from build123d import *

# Parameters (mm, degrees)
SKETCH_3_R          = 6
CUT_EXTRUDE_1_DEPTH = 1
CHAMFER_1_SIZE      = 1
CHAMFER_1_SIZE2     = 0.363970234
CHAMFER_2_SIZE      = 0.5
CHAMFER_2_SIZE2     = 0.181985117


with BuildPart() as part:
    # Эскиз1 → Повернуть1 (revolve)
    with BuildSketch(Plane.XY):
        Polygon((0, 0), (0, 5), (5, 5), (5, 0), (9, 0), (9, -3), (0, -3), align=None)
    revolve(axis=Axis((0, 0, 0), (0, 1, 0)))

    # Эскиз3 → Вырез-Вытянуть1 (cut)
    with BuildSketch(Plane.XZ.offset(3)):
        Circle(SKETCH_3_R)
    extrude(amount=-CUT_EXTRUDE_1_DEPTH, mode=Mode.SUBTRACT)

    # Фаска1
    chamfer_1_edges = [part.edges().sort_by_distance(p)[0] for p in [
        (-6, -3, 0),
    ]]
    chamfer_1_side = [part.faces().sort_by_distance(p)[0] for p in [
        (-8.745441559, -3, 0),
    ]]
    chamfer(chamfer_1_edges, length=CHAMFER_1_SIZE, length2=CHAMFER_1_SIZE2, reference=chamfer_1_side[0])

    # Фаска2
    chamfer_2_edges = [part.edges().sort_by_distance(p)[0] for p in [
        (-9, -3, 0),
    ]]
    chamfer_2_side = [part.faces().sort_by_distance(p)[0] for p in [
        (-9, -1.5, 0),
    ]]
    chamfer(chamfer_2_edges, length=CHAMFER_2_SIZE, length2=CHAMFER_2_SIZE2, reference=chamfer_2_side[0])


solid = part.part
Verification items for the finished model (mm, model axes). A direction names the side the tool comes from. Coordinates: 2 decimals unless noted, no trailing zeros. Write each loop counter-clockwise with the first axis right and the second up, starting at its lowest first coordinate (ties: lowest second). Pieces come first, ordered by that corner, then holes. Notation, with made-up numbers: M 73.5,89 L 82.5,89 A31 ccw 82.5,122 Z; hole C 71,55 d7. An arc over 180 degrees is marked long. Use a Markdown table: item, result.
Q1. Set-up check for faces 4 (the face through (0, -2, 0)), 5 (the face through (-3, -3, -7)), 6 (the face through (-1.08, 2.46, 4.88)): record each of +Z, -Z, +X, -X, +Y, -Y from which the full face is reachable in a straight line by a thin tool's end or side.
Reply:
| item | result |
|---|---|
| face 4 | -Y |
| face 5 | +Z, -Z, +X, -X, -Y |
| face 6 | +Y |
Q2. Sectioned sample at C-C, the plane y = -1.25. Record the boundary of the cut face in (x, z).
Reply:
| item | result |
|---|---|
| outline | C 0,0 d18 |
Q3. Draft check along X on faces 1 (the face through (0, 5, 0)), 2 (the face through (-5.994, -2.322, 0.264)), 3 (the face through (-1.172, -1.268, -8.923)). Enter one of: +X half, -X half, draft (parallel to the pull), parting line (faces both ways), or undercut.
Reply:
| item | result |
|---|---|
| face 1 | draft |
| face 2 | undercut |
| face 3 | parting line |
Q4. Sectioned sample at A-A, the plane z = 0. Record the boundary of the cut face in (x, y), plus the area to 3 significant figures.
Reply:
| item | result |
|---|---|
| outline | M -9,-2.5 L -8.82,-3 L -7,-3 L -6,-2.64 L -6,-2 L 6,-2 L 6,-2.64 L 7,-3 L 8.82,-3 L 9,-2.5 L 9,0 L 5,0 L 5,5 L -5,5 L -5,0 L -9,0 Z |
| area | 91.5 mm² |
Q5. Go/stop test with flat-tipped pins: P1, Ø1, axis at y = 1, z = -3.5, coming from the +X side; P2, Ø1.5, axis at x = 6, z = 4, coming from the +Y side. Record where each tip stops, or that it passes through.
Reply:
| item | result |
|---|---|
| P1 | stops at x = 4 |
| P2 | stops at y = 0 |
Q6. Sectioned sample at B-B, the plane x = 0. Record the boundary of the cut face in (y, z).
Reply:
| item | result |
|---|---|
| outline | M -3,-8.82 L -2.5,-9 L 0,-9 L 0,-5 L 5,-5 L 5,5 L 0,5 L 0,9 L -2.5,9 L -3,8.82 L -3,7 L -2.64,6 L -2,6 L -2,-6 L -2.64,-6 L -3,-7 Z |
Q7. Sectioned sample at D-D, the plane y = 3. Record the boundary of the cut face in (x, z).
Reply:
| item | result |
|---|---|
| outline | C 0,0 d10 |
Q8. Thickness scan on line 1 (Z direction, x = 0, y = -2.1); line 2 (Y direction, x = 0, z = -4); line 3 (Y direction, x = 6.75, z = -3.5). Record the ranges inside material, lowest first.
Reply:
| item | result |
|---|---|
| line 1 | z = -9 to -6, 6 to 9 |
| line 2 | y = -2 to 5 |
| line 3 | y = -3 to 0 |
